For this review, take the finished solid that the model builds, in its own axes (mm). A direction names the side the tool comes from. Coordinates: 2 decimals unless noted, no trailing zeros. Loops run counter-clockwise (first coordinate to the right, second up) from the corner with the lowest first, then second, coordinate; pieces in that order, holes last.
```python
from build123d import *

# Parameters (mm, degrees)
SKETCH1_R           = 50
BOSS_EXTRUDE1_DEPTH = 180
SKETCH2_R           = 75
BOSS_EXTRUDE2_DEPTH = 160
SKETCH3_R           = 75
BOSS_EXTRUDE3_DEPTH = 128.18
SKETCH6_R           = 40
BOSS_EXTRUDE6_DEPTH = 300
SKETCH7_R           = 49.929591809
SKETCH7_R_2         = 30
BOSS_EXTRUDE7_DEPTH = 150


with BuildPart() as part:
    # Sketch1 → Boss-Extrude1 (new body)
    with BuildSketch(Plane.XY):
        with Locations((-700, 1796)):
            Circle(SKETCH1_R)
    extrude(amount=-BOSS_EXTRUDE1_DEPTH)

    # Sketch2 → Boss-Extrude2 (add)
    with BuildSketch(Plane(origin=(0, 0, -180), x_dir=(-1, 0, 0), z_dir=(0, 0, -1))):
        with Locations((700, 1796)):
            Circle(SKETCH2_R)
    extrude(amount=BOSS_EXTRUDE2_DEPTH)

    # Sketch3 → Boss-Extrude3 (add)
    with BuildSketch(Plane(origin=(-700, 0, 0), x_dir=(0, 0, -1), z_dir=(1, 0, 0))):
        with Locations((260, 1796)):
            Circle(SKETCH3_R)
    extrude(amount=-BOSS_EXTRUDE3_DEPTH)

    # Sketch6 → Boss-Extrude6 (add)
    with BuildSketch(Plane(origin=(0, 1795, 0), x_dir=(-1, 0, 0), z_dir=(0, 1, 0))):
        with Locations(Location((700, -260, 0), (0, 0, 314.999999875))):
            Circle(SKETCH6_R)
    extrude(amount=BOSS_EXTRUDE6_DEPTH)

    # Sketch7 → Boss-Extrude7 (add)
    with BuildSketch(Plane.XY.offset(-180)):
        with Locations((-699.911954828, 2125)):
            Circle(SKETCH7_R)
        with Locations((-699.911954828, 2125)):
            Circle(SKETCH7_R_2, mode=Mode.SUBTRACT)
    extrude(amount=-BOSS_EXTRUDE7_DEPTH)


solid = part.part
```
Q1. Consider section A-A (y = 2125). State the section outline as (x, z) points.
Q2. Consider section D-D (y = 1796). State the section outline as (x, z) points, then the cut area to 3 significant figures.
Q3. The part is to be moulded in two halves that separate along Y. For faces 1 (the face through (-828.18, 1797, -259)), 2 (the face through (-706.412, 2174.505, -253.95)), 3 (the face through (-652.31, 1811.02, -88.74)), say which applies: +Y half, -Y half, draft (parallel to the pull), parting line (faces both ways), or undercut.
Q4. Wall thickness on probe 1 along Y at (x, z) = (-702, -209); probe 2 along Y at (x, z) = (-699, -192); probe 3 along X at (y, z) = (2125, -263): over which ranges is each line inside the solid? List them lowest first.
Q5. Consider section B-B (x = -760). State the section outline as (y, z) points, then the cut area to 3 significant figures.
Q6. For pin 1 Ø10 at (x, z) = (-792, -275.5) entering from +Y; pin 2 Ø6 at (x, y) = (-713.5, 1868.5) entering from +Z; pin 3 Ø5 at (x, z) = (-657.5, -188) entering from -Y, all flat-tipped, find the tip position at first contact; note any pin that passes through.
Q7. Consider section C-C (x = -723). State the section outline as (y, z) points, then the cut area to 3 significant figures.
Q8. Machinability: for faces 4 (the face through (-625.073, 1799.298, -258.88)), 5 (the face through (-791.677, 1722.783, -243.741)), 6 (the face through (-678, 2104, -330)), which of the approach directions +Z, -Z, +X, -X, +Y, -Y give a long, thin tool a straight path to every point of the face, cutting with its end or side? Answer none if there is none.
Model answer:
1. outline: (-749.84, -330) - (-729.91, -330) - (-729.91, -180) - (-749.84, -180) - close; (-669.91, -330) - (-649.98, -330) - (-649.98, -180) - (-669.91, -180) - close
2. outline: (-828.18, -335) - (-775, -335) - (-775, -340) - (-625, -340) - (-625, -180) - (-650, -180) - (-650, 0) - (-750, 0) - (-750, -180) - (-775, -180) - (-775, -185) - (-828.18, -185) - close
2. area: 50,000 mm2
3. face 1: draft
3. face 2: undercut
3. face 3: parting line
4. probe 1: y = 1721.03 to 1870.97, 2075.11 to 2095.07, 2154.93 to 2174.89
4. probe 2: y = 1721.01 to 1870.99, 2075.08 to 2095.01, 2154.99 to 2174.92
4. probe 3: x = -749.84 to -729.91, -669.91 to -649.98
5. outline: (1751, -340) - (1841, -340) - (1841, -320) arc R75 ccw to (1841, -200) - (1841, -180) - (1751, -180) - (1751, -200) arc R75 ccw to (1751, -320) - close
5. area: 19,400 mm2
6. pin 1: stops at y = 1870.26
6. pin 2: stops at z = -180
6. pin 3: stops at y = 1732.56
7. outline: (1724.61, -340) - (1867.39, -340) - (1867.39, -292.73) - (2080.73, -292.73) - (2080.73, -330) - (2105.84, -330) - (2105.84, -180) - (2080.73, -180) - (2080.73, -227.27) - (1867.39, -227.27) - (1867.39, -180) - (1840.4, -180) - (1840.4, 0) - (1751.6, 0) - (1751.6, -180) - (1724.61, -180) - (1724.61, -237) arc R75 ccw to (1724.61, -283) - close; (2144.16, -330) - (2169.27, -330) - (2169.27, -180) - (2144.16, -180) - close
7. area: 60,400 mm2
8. face 4: none
8. face 5: -X
8. face 6: -Z, +X, -X, +Y
